Verification items for this drawing (mm, ordinates from the low corner). Round coordinates to 2 decimals unless told otherwise and drop trailing zeros. Loops run counter-clockwise (first coordinate to the right, second up) from the corner with the lowest first, then second, coordinate; pieces in that order, holes last. Notation, with made-up numbers: M 76,21 L 124,21 A14 cw 124,39 Z; hole C 4.25,87.5 d9. An arc over 180 degrees is marked long. Write item = value, one per line.
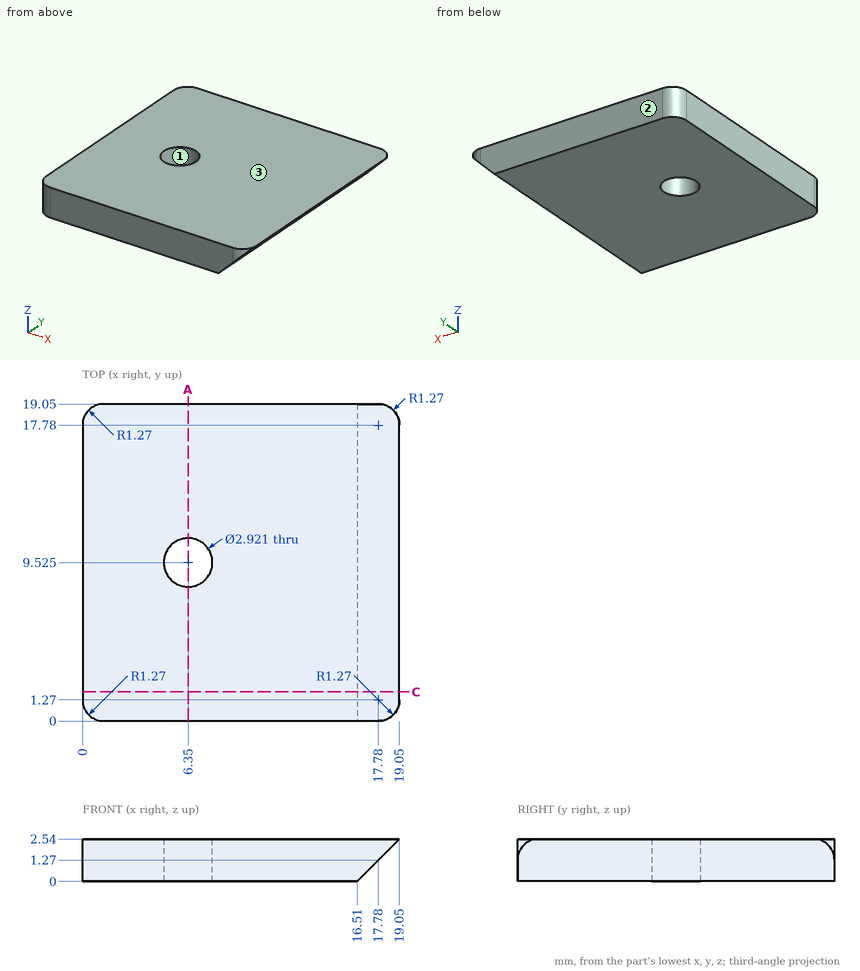
(1) Release check for a two-part mould opening along Y. For the marked faces 1, 2 and 3 record: released by +Y, released by -Y, zero draft, split by the parting line, or undercut.
Result set:
face_1 = undercut
face_2 = released by +Y
face_3 = zero draft
(2) Depth check by flat-ended pin: pin 1 Ø2.5 at (x, y) = (6.35, 9.525) entering from -Z. Enter the tip coordinate at first touch or a pass-through.
Result set:
pin_1 = through
(3) Material ranges on line 1 along Y through (x, z) = (6.35, 1.95); line 2 along X through (y, z) = (9.75, 1); line 3 along Y through (x, z) = (6, 2.25), recorded low to high. Write a range as from..to.
Result set:
line_1 = 0..8.06, 10.99..19.05
line_2 = 0..4.91, 7.79..17.51
line_3 = 0..8.11, 10.94..19.05
(4) Sectioned sample at C-C on y = 1.75. Record the cut outline in (x, z).
Result set:
outline = M 0,0 L 16.51,0 L 19.05,2.54 L 0,2.54 Z
(5) Sectioned sample at A-A on x = 6.35. Record the cut outline in (y, z).
Result set:
outline = M 0,0 L 8.06,0 L 8.06,2.54 L 0,2.54 Z; M 10.99,0 L 19.05,0 L 19.05,2.54 L 10.99,2.54 Z
